from build123d import *

# Parameters (mm, degrees)
SKETCH1_R               = 0.35
SKETCH1_R_2             = 3.25
BOSS_EXTRUDE1_DEPTH     = 1.7
CUT_EXTRUDE9_DEPTH      = 92.720556649
CUT_EXTRUDE9_DEPTH_BACK = 8
SKETCH10_R              = 1


with BuildPart() as part:
    # Sketch1 → Boss-Extrude1 (new body)
    with BuildSketch(Plane(origin=(0, 0, 0), x_dir=(0.9998727759206639, 0, 0.01595092388251767), z_dir=(0, 1, 0))):
        with BuildLine():
            Line((-2.997717637, -22.894746364), (-2.997717637, -27.430964436))
            ThreePointArc((-2.997717637, -27.430964436), (-1.503571481, -27.719382228), (0.002282363, -27.938612151))
            Line((0.002282363, -27.938612151), (0.002282363, -52.542634275))
            ThreePointArc((0.002282363, -52.542634275), (-36.656357556, -35.840573361), (-53.35841847, 0.818066557))
            Line((-53.35841847, 0.818066557), (-28.754396346, 0.818066557))
            ThreePointArc((-28.754396346, 0.818066557), (-28.535166423, -0.687787287), (-28.246748631, -2.181933443))
            Line((-28.246748631, -2.181933443), (-23.710530558, -2.181933443))
            Line((-23.710530558, -2.181933443), (-23.108601061, -2.181933443))
            ThreePointArc((-23.108601061, -2.181933443), (-15.796707511, -14.980923316), (-2.997717637, -22.292816866))
            Line((-2.997717637, -22.292816866), (-2.997717637, -22.894746364))
        make_face()
        with Locations(Location((-27.264431182, -8.755704918, 0), (0, 0, 90.913959377))):
            Circle(SKETCH1_R, mode=Mode.SUBTRACT)
        with Locations(Location((-25.368580215, -10.636127908, 0), (0, 0, 90.913959377))):
            Circle(SKETCH1_R, mode=Mode.SUBTRACT)
        with Locations(Location((-24.476362472, -13.152909386, 0), (0, 0, 90.913959377))):
            Circle(SKETCH1_R, mode=Mode.SUBTRACT)
        with Locations(Location((-24.764492621, -15.807569916, 0), (0, 0, 90.913959377))):
            Circle(SKETCH1_R, mode=Mode.SUBTRACT)
        with Locations(Location((-26.175902952, -18.074321422, 0), (0, 0, 90.913959377))):
            Circle(SKETCH1_R, mode=Mode.SUBTRACT)
        with Locations(Location((-28.431046339, -19.504205968, 0), (0, 0, 90.913959377))):
            Circle(SKETCH1_R, mode=Mode.SUBTRACT)
        with Locations(Location((-31.083263977, -19.814017383, 0), (0, 0, 90.913959377))):
            Circle(SKETCH1_R, mode=Mode.SUBTRACT)
        with Locations(Location((-33.607251635, -18.942393718, 0), (0, 0, 90.913959377))):
            Circle(SKETCH1_R, mode=Mode.SUBTRACT)
        with Locations(Location((-35.503102603, -17.061970729, 0), (0, 0, 90.913959377))):
            Circle(SKETCH1_R, mode=Mode.SUBTRACT)
        with Locations(Location((-36.395320345, -14.54518925, 0), (0, 0, 90.913959377))):
            Circle(SKETCH1_R, mode=Mode.SUBTRACT)
        with Locations(Location((-36.107190196, -11.890528721, 0), (0, 0, 90.913959377))):
            Circle(SKETCH1_R, mode=Mode.SUBTRACT)
        with Locations(Location((-34.695779865, -9.623777215, 0), (0, 0, 90.913959377))):
            Circle(SKETCH1_R, mode=Mode.SUBTRACT)
        with Locations(Location((-32.440636478, -8.193892669, 0), (0, 0, 90.913959377))):
            Circle(SKETCH1_R, mode=Mode.SUBTRACT)
        with Locations(Location((-29.78841884, -7.884081253, 0), (0, 0, 90.913959377))):
            Circle(SKETCH1_R, mode=Mode.SUBTRACT)
        with Locations(Location((-30.435841409, -13.849049318, 0), (0, 0, 90.913959377))):
            Circle(SKETCH1_R_2, mode=Mode.SUBTRACT)
    extrude(amount=BOSS_EXTRUDE1_DEPTH)

    # Sketch10 → Cut-Extrude9 (cut, two sides: drawn at the far end of the back side and taken through both)
    with BuildSketch(Plane(origin=(0, -51.287040458, 0), x_dir=(0.9998727759206634, 0, 0.015950923882551597), z_dir=(0, 1, 0)).offset(-CUT_EXTRUDE9_DEPTH_BACK)):
        with Locations(Location((-12.504691316, -31.747044129, 0), (0, 0, 270.913959377))):
            Circle(SKETCH10_R)
        with Locations(Location((-47.53974173, -5.120311842, 0), (0, 0, 270.913959377))):
            Circle(SKETCH10_R)
    extrude(amount=CUT_EXTRUDE9_DEPTH + CUT_EXTRUDE9_DEPTH_BACK, mode=Mode.SUBTRACT)


solid = part.part
Geometry: final body of the model. Coordinates: model frame, mm. Round coordinates to 2 decimals unless told otherwise and drop trailing zeros. Loops run counter-clockwise (first coordinate to the right, second up) from the corner with the lowest first, then second, coordinate; pieces in that order, holes last.
Q1. Material intervals for L1, parallel to X at y = 0.8, z = 41.5; L2, parallel to Z at x = -26, y = 0.3; L3, parallel to X at y = 1.65, z = 35, sorted ascending.
Q2. Section A-A on y = 0.7. State how many separate pieces and enclosed holes the cut face has, plus the area to 3 significant figures.
Q3. Section B-B on z = 39.5. Return loops of the section in (x, y).
Q4. Section C-C on x = -42. Return loops of the section in (y, z).
Q5. Pull-direction query (X, two-part tool) for faces 1 (the cylindrical face through (-48.503, 0.838, 4.823)), 2 (the cylindrical face through (-36.82, 0.838, 35.663)), 3 (the cylindrical face through (-16.178, 0.838, 14.577)), 4 (the flat face through (-27, 0, 25)); classes: released by +X, released by -X, zero draft, split by the parting line, or undercut.
Q6. Pin query (flat end, axial travel): P1, Ø5, axis at x = -46.5, z = 30.5, coming from the -Y side. Return the tip coordinate at first contact, or that it passes through.
Evaluation:
1. L1: x = -30.08 to -0.66
1. L2: z = 1.77 to 44.25
1. L3: x = -37.47 to -0.56
2. separate pieces: 1
2. enclosed holes: 17
2. area: 1,670 mm2
3. outline: (-32.63, 0) - (-0.63, 0) - (-0.63, 1.7) - (-32.63, 1.7) - close
4. outline: (0, -1.49) - (1.7, -1.49) - (1.7, 29.64) - (0, 29.64) - close
5. face 1: undercut
5. face 2: released by -X
5. face 3: released by +X
5. face 4: zero draft
6. P1: passes through
